The model under review builds one solid part; all positions refer to its coordinate system, in mm. A direction names the side the tool comes from. Round coordinates to 2 decimals unless told otherwise and drop trailing zeros. Order: outer loops, then holes, each group sorted by start corner. A loop starts at its lowest first (then second) coordinate and runs counter-clockwise, first axis right, second up. Notation, with made-up numbers: M 5.5,38 L 55.5,38 A19 cw 55.5,46 Z; hole C 2.5,3 d11. An arc over 180 degrees is marked long. Use a Markdown table: item, result. Add a question column.
1. Consider section B-B on x = 6.25. State the section outline as (y, z) points (1 decimal), then the cut area to 3 significant figures.
2. The part is to be moulded in two halves that separate along Z. For faces 3 (the flat face through (5, 50, -25.4)), 4 (the flat face through (6, 94.018, 25)), 5 (the flat face through (0, 17, 59)), 6 (the flat face through (6, 101.6, 25)), say which applies: +Z half, -Z half, draft (parallel to the pull), parting line (faces both ways), or undercut.
3. Consider section C-C on z = 36. State the section outline as (x, y) points, then the cut area to 3 significant figures.
4. Insertion check: P1, Ø5, axis at y = 86, z = -6, coming from the +X side; P2, Ø12, axis at y = 80, z = 9, coming from the -X side. Each pin has a flat end and moves straight along its axis. Give the tip position at first contact, or say it passes through.
5. Consider section A-A on y = 84. State the section outline as (x, z) points (1 decimal), then the cut area to 3 significant figures.
6. For faces 1 (the flat face through (6, 7.582, -9)), 2 (the flat face through (5, 0, 63)), list the 3-axis set-ups (+Z, -Z, +X, -X, +Y, -Y) from which the entire face can be reached by the end or side of a thin tool; tool diameter is ignored.
7. To check wall thickness, follow probe 1 along Z at (x, y) = (4.75, 21.5) (1 decimal); probe 2 along Y at (x, z) = (12, 59); probe 3 along Y at (x, z) = (8.5, 2). State the ranges of each line that lie inside material, in increasing order.
8. Consider section D-D on y = 58. State the section outline as (x, z) points (1 decimal), then the cut area to 3 significant figures.
Autodesk Inventor part; units mm, degrees
ref_plane "YZ Plane" through (0, 0, 0) normal (1, 0, 0) x (0, 1, 0)
ref_plane "XZ Plane" through (0, 0, 0) normal (0, 1, 0) x (-1, 0, 0)
ref_plane "XY Plane" through (0, 0, 0) normal (0, 0, 1) x (1, 0, 0)
sketch "Sketch3" plane through (0, 0, 0) normal (1, 0, 0) x (0, 1, 0)
  line L0 (0, 0) -> (25.4, 0)
  line L1 (25.4, 0) -> (25.4, -25.4)
  line L2 (25.4, -25.4) -> (0, -25.4)
  line L3 (0, -25.4) -> (0, 0)
  line L4 (25.4, -23.8125) -> (1.5875, -23.8125)
  line L5 (1.5875, -23.8125) -> (1.5875, 0)
  line L6 (7.5819, -17.8125) -> (25.4, -17.8125)
  line L7 (7.5819, 0) -> (7.5819, -17.8125)
  line L8 (9.1694, 1) -> (9.1694, -16.225)
  line L9 (9.1694, -16.225) -> (25.4, -16.225)
  point P0 (25.4, -16.225)
  point P1 (9.1694, 0)
  dimension "d15" = 25.4
  dimension "d16" = 25.4
  dimension "d17" = 1.5875
  dimension "d18" = 6
  dimension "d19" = 1.5875
  dimension "d24" = 5.9944
extrude "Extrusion3" add sketch "Sketch3" along normal blind 25.4 contours L0 L5 L4 L1 L2 L3 | L0 L8 L9 L1 L6 L7
sketch "Sketch4" plane through (0, 0, 0) normal (-1, 0, 0) x (0, 0, 1)
  line L0 (-25.4, 0) -> (-25.4, 25.4)
  line L1 (-25.4, 25.4) -> (0, 25.4)
  line L2 (0, 25.4) -> (0, 0)
  line L3 (0, 0) -> (-25.4, 0)
  line L4 (-25.4, 0) -> (-25.4, 25.4)
extrude "Extrusion4" add sketch "Sketch4" along normal blind 1.5875
sketch "Sketch5" plane through (25.4, 7.5819, 0) normal (0, 0, 1) x (1, 0, 0)
  line L0 (-25.4, 0) -> (0, 0)
  line L1 (0, 1.5875) -> (0, 0)
  line L2 (-25.4, 1.5875) -> (0, 1.5875)
  line L3 (-25.4, 1.5875) -> (-25.4, 17.8181)
  line L4 (-25.4, 17.8181) -> (-26.9875, 17.8181)
  line L5 (-26.9875, -7.5819) -> (-26.9875, 17.8181)
  line L6 (-26.9875, -7.5819) -> (0, -7.5819)
  line L7 (0, -5.9944) -> (0, -7.5819)
  line L8 (-25.4, -5.9944) -> (0, -5.9944)
  line L9 (-25.4, -5.9944) -> (-25.4, 0)
  line L10 (-26.9875, 1.5875) -> (-25.4, 1.5875)
  point P0 (-25.4, -7.5819)
extrude "Extrusion5" add sketch "Sketch5" along normal blind 25.4 contours L9 L8 L7 L6 L5 L10 L2 L1 L0
sketch "Sketch6" plane through (25.4, 25.4, -16.225) normal (0, 1, 0) x (1, 0, 0)
  line L0 (-25.4, 0) -> (0, 0)
  line L1 (0, 1.5875) -> (0, 0)
  line L2 (-25.4, 1.5875) -> (0, 1.5875)
  line L3 (-25.4, 1.5875) -> (-25.4, 7.5875)
  line L4 (-25.4, 7.5875) -> (0, 7.5875)
  line L5 (0, 9.175) -> (0, 7.5875)
  line L6 (-26.9875, 9.175) -> (0, 9.175)
  line L7 (-26.9875, -16.225) -> (-26.9875, 9.175)
  line L8 (-25.4, -16.225) -> (-26.9875, -16.225)
  line L9 (-25.4, -16.225) -> (-25.4, 0)
  line L10 (-26.9875, 0) -> (-25.4, 0)
  point P0 (-25.4, -16.225)
extrude "Extrusion6" add sketch "Sketch6" along normal blind 25.4 contours L10 L7 L6 L5 L4 L3 L2 L1 L0
mirror "Mirror1" about plane through (11.9062, 4.5847, 25.4) normal (0, 0, 1)
mirror "Mirror2" about plane through (11.9062, 50.8, -20.8125) normal (0, 1, 0)
sketch "Sketch7" plane through (-1.5875, 0, 76.2) normal (0, 0, 1) x (1, 0, 0)
  line L0 (26.9875, 0) -> (0, 0)
  line L1 (26.9875, 0) -> (14.2875, 0)
  line L2 (14.2875, 0) -> (14.2875, 107.076)
  line L3 (14.2875, 107.076) -> (26.9875, 107.076)
  line L4 (26.9875, 107.076) -> (26.9875, 0)
  point P0 (1.5875, 0)
  dimension "d29" = 12.7
extrude "Extrusion7" cut sketch "Sketch7" against normal blind 161.925
sketch "Sketch8" plane through (-1.5875, 0, 0) normal (-1, 0, 0) x (0, 0, 1)
  line L0 (0, 9.1694) -> (50.8, 9.1694)
  line L1 (0, 9.1694) -> (50.8, 9.1694)
  line L2 (50.8, 9.1694) -> (50.8, -7.9488)
  line L3 (50.8, -7.9488) -> (0, -7.9488)
  line L4 (0, -7.9488) -> (0, 9.1694)
  point P0 (0, 0)
extrude "Extrusion8" cut sketch "Sketch8" against normal blind 161.925
properties part number "end cap"
Answer block:
| question | item | result |
|---|---|---|
| 1 | outline | M 0,-25.4 L 101.6,-25.4 L 101.6,76.2 L 0,76.2 L 0,50.8 L 1.6,50.8 L 1.6,74.6 L 100,74.6 L 100,-23.8 L 1.6,-23.8 L 1.6,0 L 0,0 Z; M 7.6,-17.8 L 94,-17.8 L 94,68.6 L 7.6,68.6 L 7.6,50.8 L 9.2,50.8 L 9.2,67 L 92.4,67 L 92.4,-16.2 L 9.2,-16.2 L 9.2,0 L 7.6,0 Z |
| 1 | area | 1,010 mm^2 |
| 2 | face 3 | -Z half |
| 2 | face 4 | undercut |
| 2 | face 5 | undercut |
| 2 | face 6 | draft |
| 3 | outline | M -1.59,92.43 L 12.7,92.43 L 12.7,94.02 L 0,94.02 L 0,100.01 L 12.7,100.01 L 12.7,101.6 L -1.59,101.6 Z |
| 3 | area | 54.9 mm^2 |
| 4 | P1 | x = 0 |
| 4 | P2 | through |
| 5 | outline | M -1.6,-25.4 L 12.7,-25.4 L 12.7,-23.8 L 0,-23.8 L 0,-17.8 L 12.7,-17.8 L 12.7,-16.2 L 0,-16.2 L 0,0 L -1.6,0 Z; M -1.6,50.8 L 0,50.8 L 0,67 L 12.7,67 L 12.7,68.6 L 0,68.6 L 0,74.6 L 12.7,74.6 L 12.7,76.2 L -1.6,76.2 Z |
| 5 | area | 161 mm^2 |
| 6 | face 1 | +X |
| 6 | face 2 | +Z, -Z, +X, -X, -Y |
| 7 | probe 1 | -25.4 to -23.8, -17.8 to -16.2, 67 to 68.6, 74.6 to 76.2 |
| 7 | probe 2 | 0 to 1.59, 7.58 to 9.17, 92.43 to 94.02, 100.01 to 101.6 |
| 7 | probe 3 | 92.43 to 94.02, 100.01 to 101.6 |
| 8 | outline | M -1.6,-25.4 L 12.7,-25.4 L 12.7,-23.8 L 0,-23.8 L 0,-17.8 L 12.7,-17.8 L 12.7,-16.2 L -1.6,-16.2 Z; M -1.6,67 L 12.7,67 L 12.7,68.6 L 0,68.6 L 0,74.6 L 12.7,74.6 L 12.7,76.2 L -1.6,76.2 Z |
| 8 | area | 110 mm^2 |
